Read the model definition and answer for the solid it produces. Units are mm, in the model's axes. A direction names the side the tool comes from. Round coordinates to 2 decimals unless told otherwise and drop trailing zeros. Write each loop counter-clockwise with the first axis right and the second up, starting at its lowest first coordinate (ties: lowest second). Pieces come first, ordered by that corner, then holes. Notation, with made-up numbers: (55, 38) -> (64, 38) arc R11 cw to (64, 57) -> close; hole circle Ø3 at (63.5, 19.25). An arc over 180 degrees is marked (long way). Return JSON: item names as keys, results as strings. Group by question number.
(1) The mould has two halves that part along Z. Classify faces 1 (the cylindrical face through (146.01, 47.76, -452.1)), 2 (the flat face through (146, 0, 462.763)), 3 (the cylindrical face through (146.031, 48.89, -453.215)): released by +Z, released by -Z, zero draft, split by the parting line, or undercut.
(2) A cutting plane is placed at C-C on y = 48. Give the vertices of the cut face in (x, z).
(3) Straight lines are drawn through the part: line 1 (Z direction, x = 217, y = 9); line 2 (X direction, y = 25, z = 398.5); line 3 (Z direction, x = 132.5, y = -50.5). For each, find the intervals that lie inside material, in ascending order.
(4) Given pin 1 (1.3 mm diameter, centred on y = 57, z = 182.5, fed in from +X); pin 2 (5 mm diameter, centred on x = 237, y = -38, fed in from +Z); pin 3 (4 mm diameter, centred on y = 35, z = 41, fed in from -X), each flat-ended and moving along its own axis, determine where each tip first touches the part or whether it passes through.
(5) For faces 4 (the flat face through (-80.962, 0, 6)), 5 (the flat face through (-11, -57.944, -34)), determine the directions among +Z, -Z, +X, -X, +Y, -Y from which every point of the face is accessible in a straight line to the end or side of a thin tool.
```python
from build123d import *

# Parameters (mm, degrees)
BOSS_EXTRUDE1_DEPTH = 57.94375
FILLET1_R           = 31.75
SHELL1_T            = -1.5875


with BuildPart() as part:
    # Sketch1 → Boss-Extrude1 (new body, symmetric)
    with BuildSketch(Plane(origin=(0, 0, 0), x_dir=(1, 0, 0), z_dir=(0, 1, 0))):
        Polygon((368.3, 380.2126), (0, 380.2126), (0, -380.2126), (368.3, -380.2126), (368.3, -462.7626), (-82.55, -462.7626), (-82.55, 462.7626), (368.3, 462.7626), align=None)
    extrude(amount=BOSS_EXTRUDE1_DEPTH, both=True)

    # Fillet1
    fillet1_edges = [part.edges().sort_by_distance(p)[0] for p in [
        (142.875, -57.94375, 462.7626),
        (-82.55, -57.94375, 0),
        (142.875, -57.94375, -462.7626),
        (-82.55, 57.94375, 0),
        (142.875, 57.94375, 462.7626),
        (142.875, 57.94375, -462.7626),
    ]]
    fillet(fillet1_edges, radius=FILLET1_R)

    # Shell1
    shell1_openings = [part.faces().sort_by_distance(p)[0] for p in [
        (184.15, 0, -380.2126),
        (0, 0, 0),
        (184.15, 0, 380.2126),
    ]]
    offset(amount=SHELL1_T, openings=shell1_openings)


solid = part.part
```
Checks:
{
 "1": {"face 1": "undercut", "face 2": "released by +Z", "face 3": "released by -Z"},
 "2": {"outline": "(-73.88, -454.09) -> (368.3, -454.09) -> (368.3, -380.21) -> (366.71, -380.21) -> (366.71, -451.85) -> (-71.64, -451.85) -> (-71.64, 451.85) -> (366.71, 451.85) -> (366.71, 380.21) -> (368.3, 380.21) -> (368.3, 454.09) -> (-73.88, 454.09) -> close"},
 "3": {"line 1": "z = -462.76 to -461.18, 461.18 to 462.76", "line 2": "x = -82.55 to -80.96, 366.71 to 368.3", "line 3": "z = -451.44 to -448.87, 448.87 to 451.44"},
 "4": {"pin 1": "stops at x = 0", "pin 2": "stops at z = 461.37", "pin 3": "stops at x = -81.81"},
 "5": {"face 4": "none", "face 5": "+Z, -Z, +X, -X, -Y"}
}
